Verification items for the finished model (mm, model axes). A direction names the side the tool comes from. Coordinates: 2 decimals unless noted, no trailing zeros. Write each loop counter-clockwise with the first axis right and the second up, starting at its lowest first coordinate (ties: lowest second). Pieces come first, ordered by that corner, then holes. Notation, with made-up numbers: (60, -11.5) -> (80, -11.5) arc R3 cw to (80, -7.5) -> close; hole circle Ø3 at (63.25, 1). An arc over 180 degrees is marked (long way). Write item = value, one per line. Start each with the question number.
(1) Section check B-B (y = 38.1). Record the cut outline in (x, z) (3 decimals), plus the area to 3 significant figures.
(2) Section check C-C (x = 70). Record the cut outline in (y, z) (3 decimals), plus the area to 3 significant figures.
(3) Material ranges on probe 1 along Y at (x, z) = (16, 0.1); probe 2 along X at (y, z) = (65.5, 1.35); probe 3 along X at (y, z) = (15, 2.3), recorded low to high. Write a range as [from, to].
(4) Mould release check, pull along X, two halves, no side actions. Record for faces 5 (the face through (59.376, 74.842, 1.61)), 6 (the face through (107.95, 25, 2)), 7 (the face through (53, 0, 2)), 8 (the face through (0.91, 0.95, 1.61)): released by +X, released by -X, zero draft, split by the parting line, or undercut.
(5) Section check A-A (y = 25.4). Record the cut outline in (x, z) (3 decimals).
(6) Section check D-D (z = 1.05). State how many separate pieces and enclosed holes the cut face has, plus the area to 3 significant figures.
(7) Set-up check for faces 1 (the face through (107, 0.91, 1.61)), 2 (the face through (100, 50.8, 2)), 3 (the face through (48.648, 74.768, 1.61)), 4 (the face through (8, 50.8, 2)): record each of +Z, -Z, +X, -X, +Y, -Y from which the full face is reachable in a straight line by a thin tool's end or side.
(8) Gauge pin test, flat ends, axial feed: pin 1 Ø1 at (y, z) = (59, 2) entering from -X; pin 2 Ø1.6 at (y, z) = (69, 2.5) entering from -X; pin 3 Ø1.6 at (x, z) = (98.5, 1.5) entering from +Y. Record the tip position at first contact, or that the pin passes through.
Autodesk Inventor part; units mm, degrees
ref_plane "YZ Plane" through (0, 0, 0) normal (1, 0, 0) x (0, 1, 0)
ref_plane "XZ Plane" through (0, 0, 0) normal (0, 1, 0) x (-1, 0, 0)
ref_plane "XY Plane" through (0, 0, 0) normal (0, 0, 1) x (1, 0, 0)
sketch "Sketch1" plane through (0, 0, 0) normal (0, 0, 1) x (1, 0, 0)
  line L0 (0, 0) -> (107.95, 0)
  line L1 (107.95, 0) -> (107.95, 50.8)
  line L2 (107.95, 50.8) -> (92.075, 50.8)
  line L3 (92.075, 50.8) -> (83.3438, 76.2)
  line L4 (83.3438, 76.2) -> (57.9438, 76.2)
  line L5 (57.9438, 76.2) -> (57.9438, 63.5)
  line L6 (50.0063, 63.5) -> (50.0063, 76.2)
  line L7 (50.0063, 76.2) -> (24.6062, 76.2)
  line L8 (24.6062, 76.2) -> (15.875, 50.8)
  line L9 (15.875, 50.8) -> (0, 50.8)
  line L10 (0, 50.8) -> (0, 0)
  circle A0 centre (53.975, 25.4) radius 2.5019
  circle A1 centre (15.875, 38.1) radius 2.5019
  circle A2 centre (15.875, 12.7) radius 2.5019
  circle A3 centre (92.075, 38.1) radius 2.5019
  circle A4 centre (92.075, 12.7) radius 2.5019
  arc A5 (50.0063, 63.5) -> (57.9438, 63.5) centre (53.975, 63.5) ccw
  circle A6 centre (37.3063, 63.5) radius 2.3813
  circle A7 centre (70.6437, 63.5) radius 2.3813
  dimension "d0" = 50.8
  dimension "d1" = 107.95
  dimension "d2" = 7.9375
  dimension "d3" = 53.975
  dimension "d4" = 25.4
  dimension "d5" = 5.0038
  dimension "d6" = 38.1
  dimension "d7" = 12.7
  dimension "d8" = 25.4
  dimension "d9" = 38.1
  dimension "d11" = 25.4
  dimension "d12" = 25.4
  dimension "d14" = 12.7
  dimension "d15" = 4.7625
  dimension "d16" = 4.7625
  dimension "d17" = 12.7
  dimension "d18" = 12.7
extrude "Extrusion1" add sketch "Sketch1" along normal blind 3.175
fillet "Fillet1" radius 3.175 8 edges at (15.875, 50.8, 1.5875) (0, 50.8, 1.5875) (0, 0, 1.5875) (107.95, 0, 1.5875) (107.95, 50.8, 1.5875) (92.075, 50.8, 1.5875) (83.3438, 76.2, 1.5875) (24.6062, 76.2, 1.5875)
fillet "Fillet2" radius 4.7625 2 edges at (50.0063, 76.2, 1.5875) (57.9438, 76.2, 1.5875)
equation "\"d16\" = d15"
properties part number "Bumper Plates"
Response:
q1.outline = (0, 0) -> (13.373, 0) -> (13.373, 3.175) -> (0, 3.175) -> close; (18.377, 0) -> (89.573, 0) -> (89.573, 3.175) -> (18.377, 3.175) -> close; (94.577, 0) -> (107.95, 0) -> (107.95, 3.175) -> (94.577, 3.175) -> close
q1.area = 311 mm2
q2.outline = (0, 0) -> (61.207, 0) -> (61.207, 3.175) -> (0, 3.175) -> close; (65.793, 0) -> (76.2, 0) -> (76.2, 3.175) -> (65.793, 3.175) -> close
q2.area = 227 mm2
q3.probe_1 = [0, 10.2], [15.2, 35.6], [40.6, 51.89]
q3.probe_2 = [20.93, 36.01], [38.6, 50.01], [57.94, 69.35], [71.94, 87.02]
q3.probe_3 = [0, 14.89], [16.86, 91.09], [93.06, 107.95]
q4.face_5 = undercut
q4.face_6 = released by +X
q4.face_7 = zero draft
q4.face_8 = released by -X
q5.outline = (0, 0) -> (51.473, 0) -> (51.473, 3.175) -> (0, 3.175) -> close; (56.477, 0) -> (107.95, 0) -> (107.95, 3.175) -> (56.477, 3.175) -> close
q6.separate_pieces = 1
q6.enclosed_holes = 7
q6.area = 6,920 mm2
q7.face_1 = +Z, -Z, +X, -Y
q7.face_2 = +Z, -Z, +X, +Y
q7.face_3 = +Z, -Z, +Y
q7.face_4 = +Z, -Z, -X, +Y
q8.pin_1 = 18.52
q8.pin_2 = 21.86
q8.pin_3 = 50.8
